Geometry check sheet. Reference: the model listing, model coordinates, mm. A direction names the side the tool comes from. Coordinates: 2 decimals unless noted, no trailing zeros. Order: outer loops, then holes, each group sorted by start corner. A loop starts at its lowest first (then second) coordinate and runs counter-clockwise, first axis right, second up. Notation, with made-up numbers: M -7,71 L 8,71 A32 ccw 8,106 Z; hole C 35,0 d1. An arc over 180 degrees is marked long. One line per item, written item: value. Start each with the question number.
1) Go/stop test with flat-tipped pins: P1, Ø3.5, axis at x = 1.5, y = 9, coming from the -Z side; P2, Ø10, axis at x = 31.75, z = 90.49, coming from the -Y side; P3, Ø1.6, axis at x = 1.5, y = 16, coming from the +Z side. Record where each tip stops, or that it passes through.
2) Thickness scan on L1, parallel to Y at x = 52.5, z = 6 (3 decimals); L2, parallel to X at y = 22, z = 31.5 (3 decimals); L3, parallel to X at y = 24.25, z = 92.5. Record the ranges inside material, lowest first. Write a range as from..to.
3) Sectioned sample at B-B, the plane y = 13. Enter the section's corners in (x, z) (3 decimals).
4) Draft check along X on faces 1 (the flat face through (63.5, 13, 63)), 2 (the flat face through (31, 24, 127)), 3 (the cylindrical face through (32.029, 1.61, 84.144)). Enter one of: pulls with the +X half, pulls with the -X half, needs draft (parallel to the pull), parting line crosses it, or undercut.
5) Sectioned sample at C-C, the plane z = 53.5. Enter the section's corners in (x, y) (3 decimals).
6) Sectioned sample at D-D, the plane x = 31.75. Enter the section's corners in (y, z) (1 decimal), then the cut area to 3 significant figures.
7) Sectioned sample at A-A, the plane x = 19. Enter the section's corners in (y, z) (3 decimals).
8) Access from +Z, -Z, +X, -X, +Y, -Y to the whole of each face (thin tool, end or side, straight path). Record for faces 4 (the flat face through (31, 2, 0)), 5 (the flat face through (31, 2, 127)), 6 (the flat face through (2, 13, 19.05)), 7 (the flat face through (3.175, 13, 63)), 8 (the flat face through (2, 13, 107.95)).
```python
from build123d import *

# Parameters (mm, degrees)
SKETCH1_W           = 63.5
SKETCH1_H           = 25.4
SKETCH1_W_2         = 57.15
SKETCH1_H_2         = 19.05
EXTRUDE_THIN1_DEPTH = 127
SKETCH2_W           = 19.05
SKETCH2_H           = 19.05
CUT_EXTRUDE1_DEPTH  = 145.244271983
SKETCH3_W           = 19.05
SKETCH3_H           = 19.05
CUT_EXTRUDE2_DEPTH  = 145.244271983
SKETCH4_R           = 6.35
CUT_EXTRUDE3_DEPTH  = 145.244271983


with BuildPart() as part:
    # Sketch1 → Extrude-Thin1 (new body)
    with BuildSketch(Plane.XY):
        with Locations((31.75, 12.7)):
            Rectangle(SKETCH1_W, SKETCH1_H)
        with Locations((31.75, 12.7)):
            Rectangle(SKETCH1_W_2, SKETCH1_H_2, mode=Mode.SUBTRACT)
    extrude(amount=EXTRUDE_THIN1_DEPTH)

    # Sketch2 → Cut-Extrude1 (cut, through all)
    with BuildSketch(Plane(origin=(63.5, 0, 0), x_dir=(0, 0, -1), z_dir=(1, 0, 0))):
        with Locations((-9.525, 12.7)):
            Rectangle(SKETCH2_W, SKETCH2_H)
    extrude(amount=-CUT_EXTRUDE1_DEPTH, mode=Mode.SUBTRACT)

    # Sketch3 → Cut-Extrude2 (cut, through all)
    with BuildSketch(Plane(origin=(63.5, 0, 0), x_dir=(0, 0, -1), z_dir=(1, 0, 0))):
        with Locations((-117.475, 12.7)):
            Rectangle(SKETCH3_W, SKETCH3_H)
    extrude(amount=-CUT_EXTRUDE2_DEPTH, mode=Mode.SUBTRACT)

    # Sketch4 → Cut-Extrude3 (cut, through all)
    with BuildSketch(Plane(origin=(0, 25.4, 0), x_dir=(1, 0, 0), z_dir=(0, 1, 0))):
        with Locations(Location((31.75, -90.4875, 0), (0, 0, 270))):
            Circle(SKETCH4_R)
    extrude(amount=-CUT_EXTRUDE3_DEPTH, mode=Mode.SUBTRACT)


solid = part.part
```
Final values:
1. P1: stops at z = 19.05
1. P2: passes through
1. P3: stops at z = 107.95
2. L1: y = 0..3.175, 22.225..25.4
2. L2: x = 0..3.175, 60.325..63.5
2. L3: x = 0..25.73, 37.77..63.5
3. outline: M 0,19.05 L 3.175,19.05 L 3.175,107.95 L 0,107.95 Z; M 60.325,19.05 L 63.5,19.05 L 63.5,107.95 L 60.325,107.95 Z
4. face 1: pulls with the +X half
4. face 2: needs draft
4. face 3: undercut
5. outline: M 0,0 L 63.5,0 L 63.5,25.4 L 0,25.4 Z; hole M 3.175,3.175 L 60.325,3.175 L 60.325,22.225 L 3.175,22.225 Z
6. outline: M 0,0 L 3.2,0 L 3.2,84.1 L 0,84.1 Z; M 0,96.8 L 3.2,96.8 L 3.2,127 L 0,127 Z; M 22.2,0 L 25.4,0 L 25.4,84.1 L 22.2,84.1 Z; M 22.2,96.8 L 25.4,96.8 L 25.4,127 L 22.2,127 Z
6. area: 726 mm^2
7. outline: M 0,0 L 3.175,0 L 3.175,127 L 0,127 Z; M 22.225,0 L 25.4,0 L 25.4,127 L 22.225,127 Z
8. face 4: -Z, +X, -X, +Y, -Y
8. face 5: +Z, +X, -X, +Y, -Y
8. face 6: -Z, +X, -X
8. face 7: +Z, -Z
8. face 8: +Z, +X, -X
